Autodesk Inventor part; units mm, degrees
ref_plane "YZ Plane" through (0, 0, 0) normal (1, 0, 0) x (0, 1, 0)
ref_plane "XZ Plane" through (0, 0, 0) normal (0, 1, 0) x (-1, 0, 0)
ref_plane "XY Plane" through (0, 0, 0) normal (0, 0, 1) x (1, 0, 0)
sketch "Sketch1" plane through (0, 0, 0) normal (0, 1, 0) x (-1, 0, 0)
  line L0 (16.15, 16.15) -> (-16.15, 16.15)
  line L1 (-16.15, 16.15) -> (-16.15, -16.15)
  line L2 (-16.15, -16.15) -> (16.15, -16.15)
  line L3 (16.15, -16.15) -> (16.15, 16.15)
  line L4 (16.15, 16.15) -> (-16.15, -16.15) construction
  line L5 (-16.15, 16.15) -> (16.15, -16.15) construction
  arc A0 (16.15, 13) -> (13, 16.15) centre (13, 13) ccw
  arc A1 (-13, 16.15) -> (-16.15, 13) centre (-13, 13) ccw
  arc A2 (-16.15, -13) -> (-13, -16.15) centre (-13, -13) ccw
  arc A3 (13, -16.15) -> (16.15, -13) centre (13, -13) ccw
  point P0 (0, 0)
  point P1 (13, -16.15)
  point P2 (16.15, -13)
  point P3 (-13, 16.15)
  point P4 (-16.15, 13)
  point P5 (-16.15, -13)
  point P6 (-13, -16.15)
  dimension "d0" = 32.3
  dimension "d1" = 3.15
  dimension "d4" = 360
extrude "Extrusion1" add sketch "Sketch1" along normal blind 7 contours A0 L3 A3 L2 A2 L1 A1 L0
sketch "Sketch2" plane through (0, 7, 0) normal (0, 1, 0) x (1, 0, 0)
  line L0 (-16.15, 13) -> (-16.15, -13)
  arc A0 (-16.15, -13) -> (-13, -16.15) centre (-13, -13) ccw
  line L1 (-13, -16.15) -> (13, -16.15)
  arc A1 (13, -16.15) -> (16.15, -13) centre (13, -13) ccw
  line L2 (16.15, -13) -> (16.15, 13)
  arc A2 (16.15, 13) -> (13, 16.15) centre (13, 13) ccw
  line L3 (13, 16.15) -> (-13, 16.15)
  arc A3 (-13, 16.15) -> (-16.15, 13) centre (-13, 13) ccw
  line L4 (16.15, -10.025) -> (11.1, -10.025)
  line L5 (11.1, -10.025) -> (11.1, 10.025)
  line L6 (11.1, 10.025) -> (16.15, 10.025)
  line L7 (16.15, 0) -> (11.5552, 0) construction
  point P0 (0, 0)
  point P1 (13.625, -10.025)
  point P2 (11.1, 0)
  dimension "d8" = 5.05
  dimension "d10" = 20.05
extrude "Extrusion2" cut sketch "Sketch2" against normal through all contours L2 L4 L5 L6
sketch "Sketch4" plane through (0, 0, 0) normal (0, -1, 0) x (1, 0, 0)
  line L0 (16.15, -10.025) -> (16.15, -13)
  arc A0 (13, -16.15) -> (16.15, -13) centre (13, -13) ccw
  line L1 (13, -16.15) -> (-13, -16.15)
  line L2 (16.15, 13) -> (16.15, 10.025)
  arc A1 (16.15, 13) -> (13, 16.15) centre (13, 13) ccw
  line L3 (-13, 16.15) -> (13, 16.15)
  arc A2 (-13, 16.15) -> (-16.15, 13) centre (-13, 13) ccw
  line L4 (-16.15, -13) -> (-16.15, 13)
  arc A3 (-16.15, -13) -> (-13, -16.15) centre (-13, -13) ccw
  line L5 (16.15, 13) -> (16.15, 10.025)
  arc A4 (14.95, 13) -> (13, 14.95) centre (13, 13) ccw
  line L6 (13, 14.95) -> (-13, 14.95)
  arc A5 (-13, 14.95) -> (-14.95, 13) centre (-13, 13) ccw
  line L7 (-14.95, 13) -> (-14.95, -13)
  arc A6 (-14.95, -13) -> (-13, -14.95) centre (-13, -13) ccw
  line L8 (-13, -14.95) -> (13, -14.95)
  arc A7 (13, -14.95) -> (14.95, -13) centre (13, -13) ccw
  line L9 (14.95, -13) -> (14.95, -10.025)
  line L10 (14.95, 13) -> (14.95, -10.025)
  point P0 (0, 0)
  dimension "d13" = 1.2
extrude "Extrusion3" cut sketch "Sketch4" against normal blind 6
sketch "Sketch5" plane through (0, 0, 0) normal (0, -1, 0) x (1, 0, 0)
  line L0 (14.95, 13) -> (14.95, 10.025)
  line L1 (14.95, 10.025) -> (16.15, 10.025)
  line L2 (16.15, 13) -> (16.15, 10.025)
  arc A0 (16.15, 13) -> (13, 16.15) centre (13, 13) ccw
  line L3 (-13, 16.15) -> (13, 16.15)
  arc A1 (-13, 16.15) -> (-16.15, 13) centre (-13, 13) ccw
  line L4 (-16.15, -13) -> (-16.15, 13)
  arc A2 (-16.15, -13) -> (-13, -16.15) centre (-13, -13) ccw
  line L5 (13, -16.15) -> (-13, -16.15)
  arc A3 (13, -16.15) -> (16.15, -13) centre (13, -13) ccw
  line L6 (16.15, -10.025) -> (16.15, -13)
  line L7 (16.15, -10.025) -> (14.95, -10.025)
  line L8 (14.95, -10.025) -> (14.95, -13)
  arc A4 (13, -14.95) -> (14.95, -13) centre (13, -13) ccw
  line L9 (13, -14.95) -> (-13, -14.95)
  arc A5 (-14.95, -13) -> (-13, -14.95) centre (-13, -13) ccw
  line L10 (-14.95, -13) -> (-14.95, 13)
  arc A6 (-13, 14.95) -> (-14.95, 13) centre (-13, 13) ccw
  line L11 (-13, 14.95) -> (13, 14.95)
  arc A7 (14.95, 13) -> (13, 14.95) centre (13, 13) ccw
  line L12 (-9.65, -16.15) -> (-9.65, -14.95)
  line L13 (9.55, -16.15) -> (9.55, -14.95)
  line L14 (-9.35, 14.95) -> (-9.35, 16.15)
  line L15 (8.95, 14.95) -> (8.95, 16.15)
  line L16 (-14.95, -9.175) -> (-16.15, -9.175)
  line L17 (-14.95, 0) -> (-14.0185, 0) construction
  line L18 (-14.95, 9.175) -> (-16.15, 9.175)
  point P0 (0, 0)
  dimension "d16" = 6.5
  dimension "d17" = 19.2
  dimension "d18" = 6.8
  dimension "d19" = 18.3
  dimension "d20" = 18.35
extrude "Extrusion4" cut sketch "Sketch5" against normal blind 4.4 contours L11 L14 L3 L15 | L10 L16 L4 L18 | L9 L13 L5 L12
sketch "Sketch6" plane through (0, 6, 0) normal (0, -1, 0) x (1, 0, 0)
  line L0 (8.95, 16.15) -> (8.95, 14.95)
  line L1 (-9.35, 14.95) -> (-9.35, 16.15)
  line L2 (-16.15, 9.175) -> (-14.95, 9.175)
  line L3 (-16.15, -13) -> (-16.15, 13)
  line L4 (13, -16.15) -> (-13, -16.15)
  line L5 (-16.15, 0) -> (-5.5986, 0) construction
  line L6 (0, -16.15) -> (0, -5.693) construction
  circle A0 centre (13, 13) radius 2.75
  circle A1 centre (13, -13) radius 2.75
  circle A2 centre (-13, 13) radius 2.75
  circle A3 centre (-13, -13) radius 2.75
  line L7 (11.1, -10.025) -> (16.15, -10.025)
  line L8 (16.15, -10.025) -> (16.15, -13)
  arc A4 (13, -16.15) -> (16.15, -13) centre (13, -13) ccw
  line L9 (13, -16.15) -> (-13, -16.15)
  arc A5 (-16.15, -13) -> (-13, -16.15) centre (-13, -13) ccw
  line L10 (-16.15, -13) -> (-16.15, 13)
  arc A6 (-13, 16.15) -> (-16.15, 13) centre (-13, 13) ccw
  line L11 (-13, 16.15) -> (13, 16.15)
  arc A7 (16.15, 13) -> (13, 16.15) centre (13, 13) ccw
  line L12 (16.15, 13) -> (16.15, 10.025)
  line L13 (16.15, 10.025) -> (11.1, 10.025)
  line L14 (11.1, 10.025) -> (11.1, -10.025)
  line L15 (-10.25, -16.15) -> (-10.25, -13)
  line L16 (-13, -10.25) -> (-16.15, -10.25)
  line L17 (13, -10.25) -> (16.15, -10.25)
  line L18 (10.25, -13) -> (10.25, -16.15)
  line L19 (13, 10.25) -> (16.15, 10.25)
  line L20 (10.25, 13) -> (10.25, 16.15)
  line L21 (-10.25, 13) -> (-10.25, 16.15)
  line L22 (-13, 10.25) -> (-16.15, 10.25)
  line L23 (14.95, 10.025) -> (11.1, 10.025)
  line L24 (14.95, 13) -> (14.95, 10.025)
  arc A8 (14.95, 13) -> (13, 14.95) centre (13, 13) ccw
  line L25 (-13, 14.95) -> (13, 14.95)
  arc A9 (-13, 14.95) -> (-14.95, 13) centre (-13, 13) ccw
  line L26 (-14.95, -13) -> (-14.95, 13)
  arc A10 (-14.95, -13) -> (-13, -14.95) centre (-13, -13) ccw
  line L27 (13, -14.95) -> (-13, -14.95)
  arc A11 (13, -14.95) -> (14.95, -13) centre (13, -13) ccw
  line L28 (14.95, -10.025) -> (14.95, -13)
  line L29 (11.1, -10.025) -> (14.95, -10.025)
  line L30 (11.1, 10.025) -> (11.1, -10.025)
  point P0 (0, 0)
  point P1 (14.95, -10.25)
  point P2 (10.25, -14.95)
  point P3 (-14.95, -10.25)
  point P4 (-10.25, -14.95)
  point P5 (-10.25, 14.95)
  point P6 (-14.95, 10.25)
  point P7 (10.25, 14.95)
  point P8 (14.95, 10.25)
  dimension "d48" = 5.5
  dimension "d49" = 26
  dimension "d50" = 26
extrude "Extrusion5" add sketch "Sketch6" along normal up to surface (6 mm away) contours L25 A0 L20 | L21 A2 L25 | A0 L25 A8 L24 | A2 L26 A9 L25 | A0 L24 L19 | L22 L26 A2 | L16 A3 L26 | A3 L27 A10 L26 | L15 L27 A3 | L28 A1 L17 | A1 L28 A11 L27 | L18 A1 L27 picked at (13.0785, 12.9333) picked at (-13.0785, 12.9333) picked at (-12.9333, -13.0785) picked at (12.9333, -13.0785)
sketch "Sketch7" plane through (0, 0, 0) normal (0, -1, 0) x (1, 0, 0)
  circle A0 centre (13, 13) radius 1.5
  line L0 (-16.15, -13) -> (-16.15, 13)
  line L1 (13, -16.15) -> (-13, -16.15)
  line L2 (0, -16.15) -> (0, -7.7699) construction
  line L3 (-16.15, 0) -> (-9.6467, 0) construction
  circle A1 centre (13, -13) radius 1.5
  circle A2 centre (-13, 13) radius 1.5
  circle A3 centre (-13, -13) radius 1.5
  point P0 (0, 0)
  dimension "d31" = 3
  dimension "d41" = 26
  dimension "d42" = 26
extrude "Extrusion6" cut sketch "Sketch7" against normal through all
sketch "Sketch9" plane through (0, 6, 0) normal (0, -1, 0) x (1, 0, 0)
  line L0 (11.1, -10.025) -> (14.95, -10.025)
  line L1 (11.1, 10.025) -> (11.1, -10.025)
  line L2 (14.95, 10.025) -> (11.1, 10.025)
  line L3 (-10.25, 14.95) -> (10.25, 14.95)
  line L4 (-14.95, -10.25) -> (-14.95, 10.25)
  line L5 (10.25, -14.95) -> (-10.25, -14.95)
  line L6 (14.95, 10.25) -> (14.95, 10.025)
  line L7 (14.95, -10.025) -> (14.95, -10.25)
  line L8 (-10.25, -13) -> (-10.25, -14.95)
  line L9 (10.25, -14.95) -> (10.25, -13)
  arc A0 (13, -10.25) -> (10.25, -13) centre (13, -13) ccw
  line L10 (13, -10.25) -> (14.95, -10.25)
  line L11 (14.95, 10.25) -> (13, 10.25)
  arc A1 (10.25, 13) -> (13, 10.25) centre (13, 13) ccw
  line L12 (10.25, 13) -> (10.25, 14.95)
  line L13 (-10.25, 14.95) -> (-10.25, 13)
  arc A2 (-13, 10.25) -> (-10.25, 13) centre (-13, 13) ccw
  line L14 (-13, 10.25) -> (-14.95, 10.25)
  line L15 (-14.95, -10.25) -> (-13, -10.25)
  arc A3 (-10.25, -13) -> (-13, -10.25) centre (-13, -13) ccw
  point P0 (0, 0)
extrude "Extrusion8" add sketch "Sketch9" along normal blind 1.1
sketch "Sketch10" plane through (0, 7, 0) normal (0, 1, 0) x (1, 0, 0)
  circle A0 centre (-13, 13) radius 1.5
  circle A1 centre (13, 13) radius 1.5
  circle A2 centre (13, -13) radius 1.5
  circle A3 centre (-13, -13) radius 1.5
  line L0 (11.1, 10.025) -> (16.15, 10.025)
  line L1 (16.15, 10.025) -> (16.15, 13)
  arc A4 (16.15, 13) -> (13, 16.15) centre (13, 13) ccw
  line L2 (13, 16.15) -> (-13, 16.15)
  arc A5 (-13, 16.15) -> (-16.15, 13) centre (-13, 13) ccw
  line L3 (-16.15, 13) -> (-16.15, -13)
  arc A6 (-16.15, -13) -> (-13, -16.15) centre (-13, -13) ccw
  line L4 (-13, -16.15) -> (13, -16.15)
  arc A7 (13, -16.15) -> (16.15, -13) centre (13, -13) ccw
  line L5 (16.15, -13) -> (16.15, -10.025)
  line L6 (16.15, -10.025) -> (11.1, -10.025)
  line L7 (11.1, -10.025) -> (11.1, 10.025)
  point P0 (0, 0)
extrude "Extrusion9" cut sketch "Sketch10" against normal blind 0.5
sketch "Sketch11" plane through (0, 0, 0) normal (0, -1, 0) x (1, 0, 0)
  point P0 (0, 0)
chamfer "Chamfer2" distance 0.4 angle 45 9 edges at (0, 6.5, -16.15) (15.2274, 6.5, -15.2274) (16.15, 6.5, -11.5125) (-15.2274, 6.5, -15.2274) (-16.15, 6.5, 0) (-15.2274, 6.5, 15.2274) (0, 6.5, 16.15) (15.2274, 6.5, 15.2274) (16.15, 6.5, 11.5125)
properties part number "oDrive_micro_cover_3DPrint"
The model under review builds one solid part; all positions refer to its coordinate system, in mm. A direction names the side the tool comes from. Round coordinates to 2 decimals unless told otherwise and drop trailing zeros. Write each loop counter-clockwise with the first axis right and the second up, starting at its lowest first coordinate (ties: lowest second). Pieces come first, ordered by that corner, then holes. Notation, with made-up numbers: (-24.5, -19) -> (-2.5, -19) arc R29 cw to (-2.5, 19) -> close; hole circle Ø5 at (51.5, -21). An arc over 180 degrees is marked (long way). Answer as a JSON object with one key per item and string values.
1. To check wall thickness, follow line 1 along X through (y, z) = (1.75, -13). State the ranges of the line that lie inside material, in increasing order.
Results found:
{"line 1": "x = -16.15 to -14.5, -11.5 to -10.25, 10.25 to 11.5, 14.5 to 16.15"}
2. We need section A-A on x = -8. State the section outline as (y, z) points, and give its area (3 significant figures).
Results found:
{"outline": "(4.4, -16.15) -> (6.1, -16.15) -> (6.5, -15.75) -> (6.5, 15.75) -> (6.1, 16.15) -> (4.4, 16.15) -> (4.4, 14.95) -> (4.9, 14.95) -> (4.9, -14.95) -> (4.4, -14.95) -> close", "area": "52.7 mm^2"}
3. We need section C-C on y = 1.5. State how many separate pieces and enclosed holes the cut face has, and give its area (3 significant figures).
Results found:
{"separate pieces": "4", "enclosed holes": "4", "area": "103 mm^2"}
4. We need section D-D on z = 8. State the section outline as (x, y) points, and give its area (3 significant figures).
Results found:
{"outline": "(-16.15, 4.4) -> (-14.95, 4.4) -> (-14.95, 4.9) -> (11.1, 4.9) -> (11.1, 6.5) -> (-15.75, 6.5) -> (-16.15, 6.1) -> close", "area": "44.1 mm^2"}
5. Clearance check with flat-ended pins moving along their axes: pin 1 (5 mm diameter, centred on x = -2, z = 0.5, fed in from -Y); pin 2 (1.3 mm diameter, centred on y = 1.5, z = -15.5, fed in from -X); pin 3 (0.6 mm diameter, centred on y = 3.5, z = -13.5, fed in from +X); pin 4 (1.5 mm diameter, centred on y = 2, z = -4, fed in from +X). State where each tip first meets the part, or that it passes through.
Results found:
{"pin 1": "stops at y = 4.9", "pin 2": "stops at x = -15.55", "pin 3": "stops at x = 16.14", "pin 4": "passes through"}
6. Machinability: for faces 4 (the face through (-9.35, 2.2, 15.5)), 5 (the face through (15.3, 4.7, -10.025)), 6 (the face through (-11.03, 2.48, 11.08)), 7 (the face through (-15.5, 2.2, -9.175)), which of the approach directions +Z, -Z, +X, -X, +Y, -Y give a long, thin tool a straight path to every point of the face, cutting with its end or side? Answer none if there is none.
Results found:
{"face 4": "+Z, -Z, -Y", "face 5": "+X, +Y, -Y", "face 6": "-Y", "face 7": "+X, -X, -Y"}
7. We need section B-B on x = -12. State the section outline as (y, z) points.
Results found:
{"outline": "(0, -16.15) -> (6.1, -16.15) -> (6.5, -15.75) -> (6.5, -14.12) -> (0, -14.12) -> close; (0, -11.88) -> (6.5, -11.88) -> (6.5, 11.88) -> (0, 11.88) -> (0, 10.44) -> (4.9, 10.44) -> (4.9, -10.44) -> (0, -10.44) -> close; (0, 14.12) -> (6.5, 14.12) -> (6.5, 15.75) -> (6.1, 16.15) -> (0, 16.15) -> close"}
8. The part is to be moulded in two halves that separate along X. For faces 1 (the face through (0, 5, 16.15)), 2 (the face through (10.25, 2, 14)), 3 (the face through (16.15, 3, -11)), say which applies: pulls with the +X half, pulls with the -X half, needs draft (parallel to the pull), parting line crosses it, or undercut.
Results found:
{"face 1": "needs draft", "face 2": "undercut", "face 3": "pulls with the +X half"}
